The drawing under review shows one solid part. Ordinate dimensions are in mm from its lowest x, y, z. A direction names the side the tool comes from. Round coordinates to 2 decimals unless told otherwise and drop trailing zeros. Order: outer loops, then holes, each group sorted by start corner. A loop starts at its lowest first (then second) coordinate and runs counter-clockwise, first axis right, second up. Notation, with made-up numbers: M 17,42.5 L 66,42.5 A18 ccw 66,77.5 Z; hole C 68,-4.5 d9. An arc over 180 degrees is marked long. Answer as a JSON object with one key per item and string values. Group by question number.
1) Insertion check: pin 1 Ø3 at (x, y) = (81.5, 62) entering from +Z; pin 2 Ø20.5 at (y, z) = (51.5, 43) entering from +X. Each pin has a flat end and moves straight along its axis. Give the tip position at first contact, or say it passes through.
2) To check wall thickness, follow line 1 (Z direction, x = 97, y = 70); line 2 (X direction, y = 52.5, z = 37). State the ranges of each line that lie inside material, in increasing order.
3) Consider section C-C, the plane z = 39.5. Write out the cut boundary in (x, y).
4) Consider section A-A, the plane y = 57.5. Write out the cut boundary in (x, z), then the cut area to 3 significant figures.
5) Consider section B-B, the plane x = 81.5. Write out the cut boundary in (y, z), then the cut area to 3 significant figures.
6) For the marked faces 1 and 2, list the 3-axis set-ups (+Z, -Z, +X, -X, +Y, -Y) from which the entire face can be reached by the end or side of a thin tool; tool diameter is ignored.
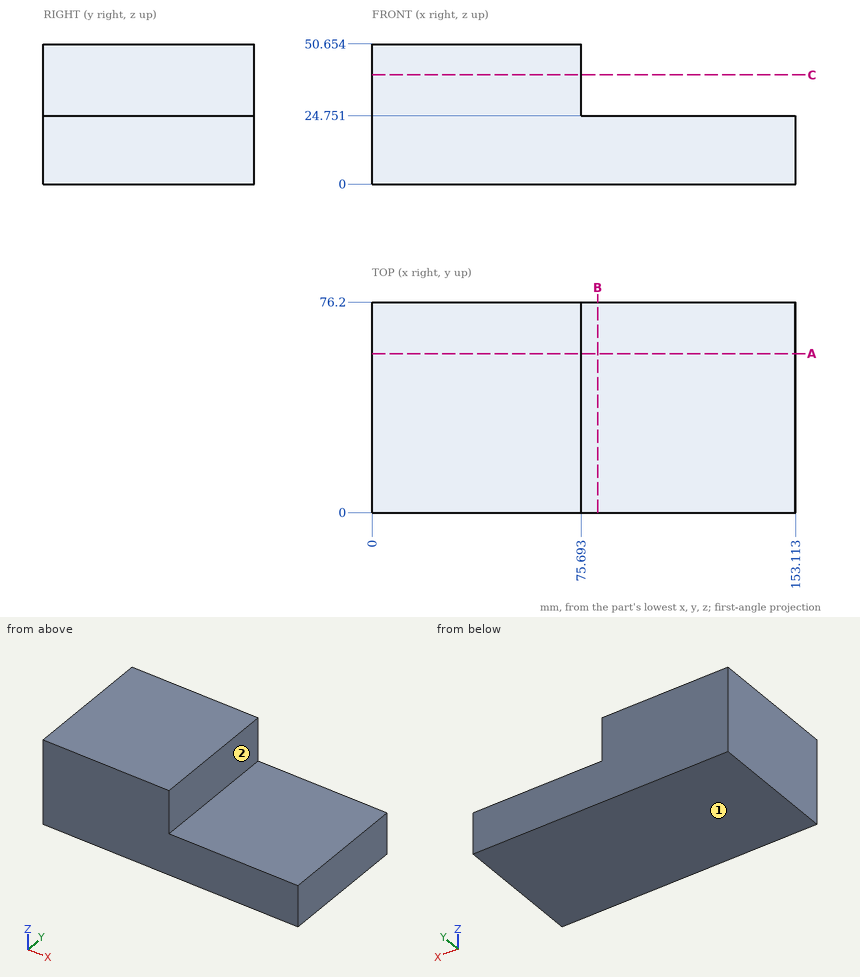
Results list:
{
 "1": {"pin 1": "z = 24.75", "pin 2": "x = 75.69"},
 "2": {"line 1": "0 to 24.75", "line 2": "0 to 75.69"},
 "3": {"outline": "M 0,0 L 75.69,0 L 75.69,76.2 L 0,76.2 Z"},
 "4": {"outline": "M 0,0 L 153.11,0 L 153.11,24.75 L 75.69,24.75 L 75.69,50.65 L 0,50.65 Z", "area": "5,750 mm^2"},
 "5": {"outline": "M 0,0 L 76.2,0 L 76.2,24.75 L 0,24.75 Z", "area": "1,890 mm^2"},
 "6": {"face 1": "-Z, +X, -X, +Y, -Y", "face 2": "+Z, +X, +Y, -Y"}
}
